The drawing under review shows one solid part. Ordinate dimensions are in mm from its lowest x, y, z. A direction names the side the tool comes from. Give positions to 0.01 mm unless a question says otherwise; leave off trailing zeros. Loops run counter-clockwise (first coordinate to the right, second up) from the corner with the lowest first, then second, coordinate; pieces in that order, holes last. Notation, with made-up numbers: M 30,58 L 82,58 A27 cw 82,88 Z; hole C 55,61.25 d10. An arc over 180 degrees is marked long. One line per item, written item: value. Start each with the question number.
Q1. To check wall thickness, follow line 1 along Z through (x, y) = (128, 14); line 2 along X through (y, z) = (10, 33) (1 decimal); line 3 along Z through (x, y) = (76.5, 13.25). State the ranges of each line that lie inside material, in increasing order. Write a range as from..to.
Q2. Mouldability with a two-part tool opening along X and no side actions: class the marked faces 3, 4 and 5 as released by +X, released by -X, zero draft, split by the parting line, or undercut.
Q3. We need section B-B on z = 45. Write out the cut boundary in (x, y) (1 decimal).
Q4. We need section A-A on y = 13.5. Write out the cut boundary in (x, z) (1 decimal).
Q5. We need section D-D on x = 112. Write out the cut boundary in (y, z).
Q6. For the marked faces 1 and 2, list the 3-axis set-ups (+Z, -Z, +X, -X, +Y, -Y) from which the entire face can be reached by the end or side of a thin tool; tool diameter is ignored.
Q7. We need section C-C on x = 77.5. Write out the cut boundary in (y, z), plus the area to 3 significant figures.
Q8. For pin 1 (8 mm diameter, centred on y = 14, z = 18, fed in from +X); pin 2 (10 mm diameter, centred on x = 19.5, z = 47, fed in from -Y); pin 3 (2 mm diameter, centred on y = 10, z = 91.5, fed in from +X); pin 4 (1 mm diameter, centred on y = 4, z = 66.5, fed in from -X), all flat-tipped, find the tip position at first contact; note any pin that passes through.
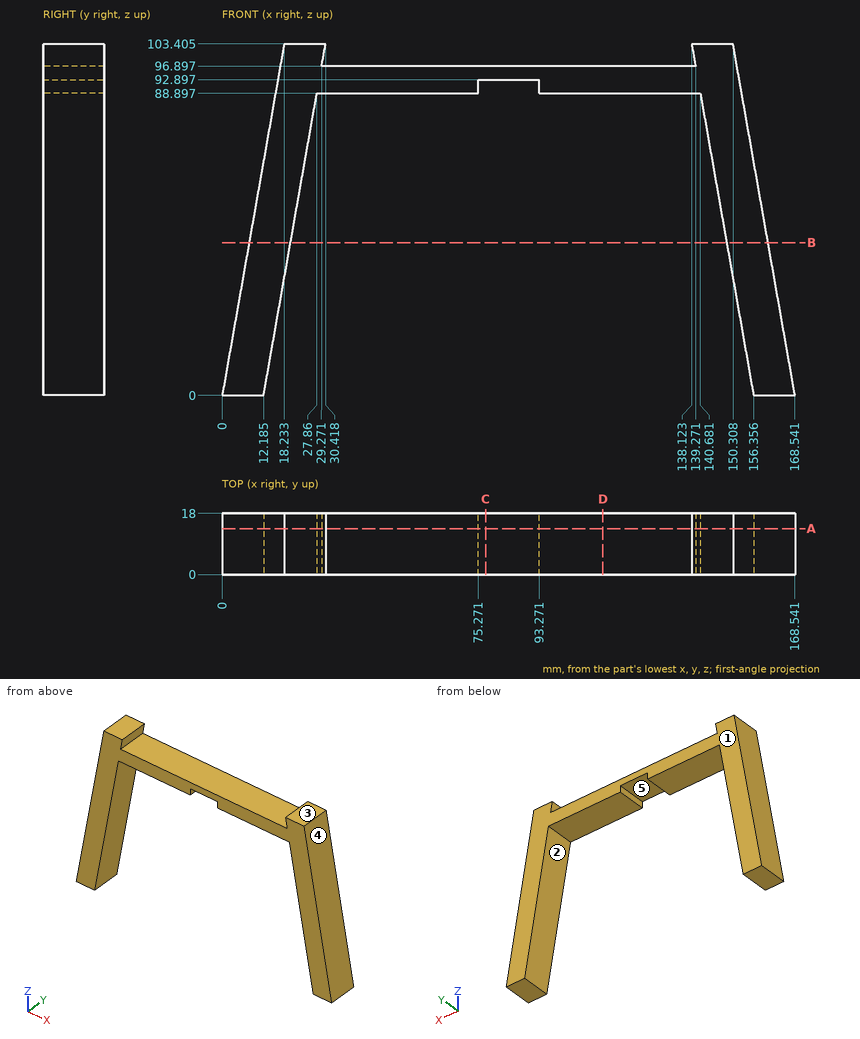
Solved:
1. line 1: 88.9..96.9
1. line 2: 5.8..18, 150.5..162.7
1. line 3: 92.9..96.9
2. face 3: zero draft
2. face 4: released by +X
2. face 5: undercut
3. outline: M 7.9,0 L 20.1,0 L 20.1,18 L 7.9,18 Z; M 148.4,0 L 160.6,0 L 160.6,18 L 148.4,18 Z
4. outline: M 0,0 L 12.2,0 L 27.9,88.9 L 75.3,88.9 L 75.3,92.9 L 93.3,92.9 L 93.3,88.9 L 140.7,88.9 L 156.4,0 L 168.5,0 L 150.3,103.4 L 138.1,103.4 L 139.3,96.9 L 29.3,96.9 L 30.4,103.4 L 18.2,103.4 Z
5. outline: M 0,88.9 L 18,88.9 L 18,96.9 L 0,96.9 Z
6. face 1: +Z, -Z, +X, -X, +Y
6. face 2: -Z, +Y, -Y
7. outline: M 0,92.9 L 18,92.9 L 18,96.9 L 0,96.9 Z
7. area: 72.0 mm2
8. pin 1: x = 166.07
8. pin 2: y = 0
8. pin 3: x = 152.58
8. pin 4: x = 11.64
